Input: part model. Units: mm. Frame: model coordinates. Face numbers are marked on the shaded views. A direction names the side the tool comes from. Give positions to 0.01 mm unless a question says otherwise; leave off trailing zeros. Loops run counter-clockwise (first coordinate to the right, second up) from the corner with the lowest first, then second, coordinate; pieces in that order, holes last. Notation, with made-up numbers: (43, 73) -> (82, 73) arc R24 ccw to (82, 86) -> close; hole circle Ø7 at (52.25, 44.5). An arc over 180 degrees is marked (long way). Answer as a JSON object with one key per item and string values. Group by question number.
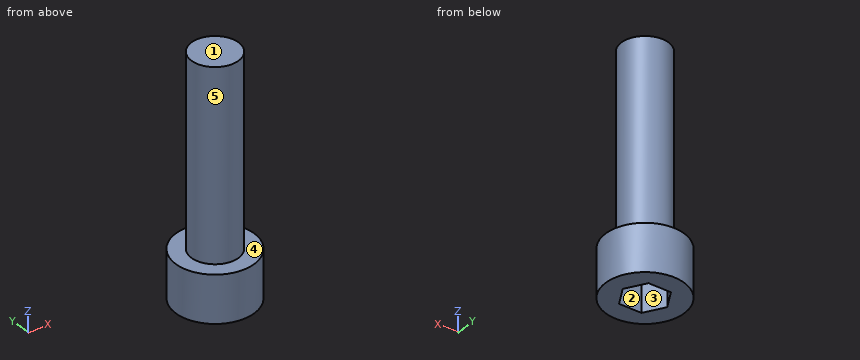
Autodesk Inventor part; units mm, degrees
ref_plane "YZ Plane" through (0, 0, 0) normal (1, 0, 0) x (0, 1, 0)
ref_plane "XZ Plane" through (0, 0, 0) normal (0, 1, 0) x (-1, 0, 0)
ref_plane "XY Plane" through (0, 0, 0) normal (0, 0, 1) x (1, 0, 0)
sketch "Sketch1" plane through (0, 0, 0) normal (0, 0, 1) x (1, 0, 0)
  circle A0 centre (0, 0) radius 5
  dimension "d0" = 10
extrude "Extrusion1" add sketch "Sketch1" along normal blind 6
sketch "Sketch2" plane through (0, 0, 6) normal (0, 0, 1) x (1, 0, 0)
  circle A0 centre (0, 0) radius 5
  circle A1 centre (0, 0) radius 3
  dimension "d3" = 6
extrude "Extrusion2" add sketch "Sketch2" along normal blind 24 contours A1
sketch "Sketch3" plane through (0, 0, 0) normal (0, 0, -1) x (-1, 0, 0)
  circle A0 centre (0, 0) radius 5
  line L0 (2.8868, 0) -> (1.4434, -2.5)
  line L1 (1.4434, -2.5) -> (-1.4434, -2.5)
  line L2 (-1.4434, -2.5) -> (-2.8868, 0)
  line L3 (-2.8868, 0) -> (-1.4434, 2.5)
  line L4 (-1.4434, 2.5) -> (1.4434, 2.5)
  line L5 (1.4434, 2.5) -> (2.8868, 0)
  dimension "d6" = 5
extrude "Extrusion3" cut sketch "Sketch3" against normal blind 4 contours L0 L1 L2 L3 L4 L5
thread "Thread1"
properties part number "m6x1"
Q1. Section C-C on y = 1.5. Return the cut outline in (x, z), then the cut area to 3 significant figures.
Q2. Ray query, probe 1 along Z at (x, y) = (1, 1.75); probe 2 along Z at (x, y) = (0, -4.5); probe 3 along X at (y, z) = (-2.25, 2). Return the intervals inside material, ascending.
Q3. Section D-D on z = 15.75. Return the cut outline in (x, y), then the cut area to 3 significant figures.
Q4. Pin query (flat end, axial travel): pin 1 Ø5 at (y, z) = (-3.5, 17) entering from +X; pin 2 Ø1 at (y, z) = (-2.5, 13) entering from -X; pin 3 Ø6 at (y, z) = (-3, 10.5) entering from +X. Return the tip coordinate at first contact, or that it passes through.
Q5. Set-up query: the marked faces 1 and 2. Return all of +Z, -Z, +X, -X, +Y, -Y with unobstructed straight access to the full face (end or side cutting, diameter ignored); none if empty.
Q6. Pull-direction query (X, two-part tool) for the marked faces 3, 4 and 5; classes: +X half, -X half, draft (parallel to the pull), parting line (faces both ways), or undercut.
Q7. Section B-B on x = 0. Return the cut outline in (y, z), then the cut area to 3 significant figures.
Q8. Section A-A on z = 3.25. Return the cut outline in (x, y), then the cut area to 3 significant figures.
Numbers:
{
 "1": {"outline": "(-4.77, 0) -> (-2.02, 0) -> (-2.02, 4) -> (2.02, 4) -> (2.02, 0) -> (4.77, 0) -> (4.77, 6) -> (2.6, 6) -> (2.6, 30) -> (-2.6, 30) -> (-2.6, 6) -> (-4.77, 6) -> close", "area": "166 mm²"},
 "2": {"probe 1": "z = 4 to 30", "probe 2": "z = 0 to 6", "probe 3": "x = -4.47 to -1.59, 1.59 to 4.47"},
 "3": {"outline": "circle Ø6 at (0, 0)", "area": "28.3 mm²"},
 "4": {"pin 1": "stops at x = 2.83", "pin 2": "stops at x = -2.24", "pin 3": "stops at x = 3"},
 "5": {"face 1": "+Z, +X, -X, +Y, -Y", "face 2": "-Z"},
 "6": {"face 3": "undercut", "face 4": "draft", "face 5": "parting line"},
 "7": {"outline": "(-5, 0) -> (-2.5, 0) -> (-2.5, 4) -> (2.5, 4) -> (2.5, 0) -> (5, 0) -> (5, 6) -> (3, 6) -> (3, 30) -> (-3, 30) -> (-3, 6) -> (-5, 6) -> close", "area": "184 mm²"},
 "8": {"outline": "circle Ø10 at (0, 0); hole (-2.89, 0) -> (-1.44, -2.5) -> (1.44, -2.5) -> (2.89, 0) -> (1.44, 2.5) -> (-1.44, 2.5) -> close", "area": "56.9 mm²"}
}
